```python
from build123d import *

# Parameters (mm, degrees)
SKETCH027_R             = 30
PAD006_DEPTH            = 13
SKETCH028_R             = 29
POCKET018_DEPTH         = 3.5
SKETCH029_R             = 27.5
PAD007_DEPTH            = 3.5
SKETCH031_W             = 32
SKETCH031_H             = 40
POCKET020_DEPTH         = 13
SKETCH032_W             = 5
SKETCH032_H             = 3
POCKET021_DEPTH         = 8
SKETCH033_R             = 2.25
POCKET022_DEPTH         = 20
SKETCH034_W             = 8
SKETCH034_H             = 5
POCKET023_DEPTH         = 10
SKETCH035_W             = 13.2
SKETCH035_H             = 7
POCKET024_DEPTH         = 9
SKETCH036_W             = 6.5
SKETCH036_H             = 7
POCKET025_DEPTH         = 5
SKETCH037_W             = 2
SKETCH037_H             = 13.2
PAD008_DEPTH            = 1
BODY005_PLACEMENT_ANGLE = 90


with BuildPart() as part:
    # Sketch027 → Pad006 (new body)
    with BuildSketch(Plane.XY):
        Circle(SKETCH027_R)
    extrude(amount=PAD006_DEPTH)

    # Sketch028 (on Face3 of Pad006) → Pocket018 (cut)
    with BuildSketch(Plane.XY.offset(13)):
        Circle(SKETCH028_R)
    extrude(amount=-POCKET018_DEPTH, mode=Mode.SUBTRACT)

    # Sketch029 (on Face5 of Pocket018) → Pad007 (join)
    with BuildSketch(Plane.XY.offset(9.5)):
        Circle(SKETCH029_R)
    extrude(amount=PAD007_DEPTH)

    # Sketch031 → Pocket020 (cut)
    with BuildSketch(Plane.XY.offset(13)):
        Rectangle(SKETCH031_W, SKETCH031_H)
    extrude(amount=-POCKET020_DEPTH, mode=Mode.SUBTRACT)

    # Sketch032 (on Face5 of Pocket020) → Pocket021 (cut)
    with BuildSketch(Plane(origin=(0, -20, 0), x_dir=(-1, 0, 0), z_dir=(0, 1, 0))):
        with Locations((0, 11.5)):
            Rectangle(SKETCH032_W, SKETCH032_H)
    extrude(amount=-POCKET021_DEPTH, mode=Mode.SUBTRACT)

    # Sketch033 (on Face9 of Pocket021) → Pocket022 (cut)
    with BuildSketch(Plane.XY.offset(13)):
        with Locations((-19.108778, -14.520833)):
            Circle(SKETCH033_R)
        with Locations((0, 24)):
            Circle(SKETCH033_R)
        with Locations((19.108778, -14.520833)):
            Circle(SKETCH033_R)
    extrude(amount=-POCKET022_DEPTH, mode=Mode.SUBTRACT)

    # Sketch034 (on Face2 of Pocket022) → Pocket023 (cut)
    with BuildSketch(Plane(origin=(0, 0, 0), x_dir=(1, 0, 0), z_dir=(0, 0, -1))):
        with Locations((0, 22.5)):
            Rectangle(SKETCH034_W, SKETCH034_H)
    extrude(amount=-POCKET023_DEPTH, mode=Mode.SUBTRACT)

    # Sketch035 (on Face10 of Pocket023) → Pocket024 (cut)
    with BuildSketch(Plane(origin=(16, 0, 0), x_dir=(0, -1, 0), z_dir=(-1, 0, 0))):
        with Locations((0, 3.5)):
            Rectangle(SKETCH035_W, SKETCH035_H)
    extrude(amount=-POCKET024_DEPTH, mode=Mode.SUBTRACT)

    # Sketch036 (on Face12 of Pocket024) → Pocket025 (cut)
    with BuildSketch(Plane(origin=(25, 0, 0), x_dir=(0, -1, 0), z_dir=(-1, 0, 0))):
        with Locations((0, 3.5)):
            Rectangle(SKETCH036_W, SKETCH036_H)
    extrude(amount=-POCKET025_DEPTH, mode=Mode.SUBTRACT)

    # Sketch037 (on Face7 of Pocket025) → Pad008 (join)
    with BuildSketch(Plane(origin=(0, 0, 7), x_dir=(1, 0, 0), z_dir=(0, 0, -1))):
        with Locations((17, 0)):
            Rectangle(SKETCH037_W, SKETCH037_H)
    extrude(amount=PAD008_DEPTH)


with BuildPart() as part_1:
    # Body005 placement: moved
    add(part.part.moved(Location((0, 0, 5))).rotate(Axis((0, 0, 5), (0, 0, 1)), BODY005_PLACEMENT_ANGLE))


solid = part_1.part
```
Check sheet for the modelled part. Datum: model origin and axes. Units: mm. A direction names the side the tool comes from. Round coordinates to 2 decimals unless told otherwise and drop trailing zeros. Order: outer loops, then holes, each group sorted by start corner. A loop starts at its lowest first (then second) coordinate and runs counter-clockwise, first axis right, second up. Notation, with made-up numbers: (11.5, 12.25) - (69.5, 12.25) arc R36 cw to (69.5, 46.25) - close; hole circle Ø8 at (9, 45.25). An arc over 180 degrees is marked (long way). Answer as CSV lines item,"result". Start each with the question number.
1) Section check B-B (x = 0). Record the cut outline in (y, z).
2) Draft check along X on faces 5 (the face through (25, 0, 10)), 6 (the face through (-2.2, 16.2, 18)). Enter one of: +X half, -X half, draft (parallel to the pull), parting line (faces both ways), or undercut.
3) Section check A-A (y = 0). Record the cut outline in (x, z), then the cut area to 4 significant figures.
4) Scan lines: probe 1 along X at (y, z) = (0, 17.1); probe 2 along X at (y, z) = (0, 10); probe 3 along Y at (x, z) = (-11, 14.75). Record each from-to range of solid material in increasing order.
5) Depth check by flat-ended pin: pin 1 (1.2 mm diameter, centred on x = 26, y = -1, fed in from +Z); pin 2 (4 mm diameter, centred on y = 2.5, z = 16.5, fed in from +X); pin 3 (5 mm diameter, centred on y = 11.5, z = 10.5, fed in from +X); pin 4 (4 mm diameter, centred on x = 14.52, y = -19.11, fed in from -Z). Enter the tip coordinate at first touch or a pass-through.
6) Tool access check on faces 1 (the face through (3.25, 27, 8)), 2 (the face through (5, 25, 9)), 3 (the face through (20, 9, 12)), 4 (the face through (26, 0, 15)). Record the directions out of +Z, -Z, +X, -X, +Y, -Y that give a thin tool (end or side, any length) a straight path to the whole face; none if there is none.
7) Section check D-D (z = 13.5). Record the cut outline in (x, y), then the cut area to 3 significant figures.
8) Section check C-C (z = 8.25). Record the cut outline in (x, y), then the cut area to 3 significant figures.
Determined:
1,outline,"(-30, 5) - (-16, 5) - (-16, 18) - (-27.5, 18) - (-27.5, 14.5) - (-29, 14.5) - (-29, 18) - (-30, 18) - close; (16, 11) - (18, 11) - (18, 12) - (30, 12) - (30, 18) - (29, 18) - (29, 14.5) - (27.5, 14.5) - (27.5, 18) - (16, 18) - close"
2,face 5,"undercut"
2,face 6,"draft"
3,outline,"(-30, 5) - (-26.25, 5) - (-26.25, 18) - (-27.5, 18) - (-27.5, 14.5) - (-29, 14.5) - (-29, 18) - (-30, 18) - close; (-21.75, 5) - (-20, 5) - (-20, 18) - (-21.75, 18) - close; (25, 5) - (30, 5) - (30, 18) - (29, 18) - (29, 14.5) - (27.5, 14.5) - (27.5, 15) - (25, 15) - close"
3,area,"118.5 mm^2"
4,probe 1,"-30 to -29, -27.5 to -26.25, -21.75 to -20, 29 to 30"
4,probe 2,"-30 to -26.25, -21.75 to -20, 25 to 30"
4,probe 3,"-27.91 to -26.83, -25.2 to -16, 16 to 25.2, 26.83 to 27.91"
5,pin 1,"z = 15"
5,pin 2,"x = 30"
5,pin 3,"x = 28.62"
5,pin 4,"through"
6,face 1,"-Z, +Y"
6,face 2,"-Z"
6,face 3,"+Z, -Z"
6,face 4,"+Z"
7,outline,"circle Ø60 at (0, 0); hole circle Ø4.5 at (-24, 0); hole (-20, -16) - (20, -16) - (20, -4) - (25, -4) - (25, 4) - (20, 4) - (20, 16) - (-20, 16) - close; hole circle Ø4.5 at (14.52, -19.11); hole circle Ø4.5 at (14.52, 19.11)"
7,area,"1,460 mm^2"
8,outline,"(-20, -16) - (-20, 16) - (-6.6, 16) - (-6.6, 25) - (-3.25, 25) - (-3.25, 29.82) arc R30 ccw (long way) to (3.25, 29.82) - (3.25, 25) - (6.6, 25) - (6.6, 16) - (20, 16) - (20, 4) - (25, 4) - (25, -4) - (20, -4) - (20, -16) - close; hole circle Ø4.5 at (-24, 0); hole circle Ø4.5 at (14.52, -19.11); hole circle Ø4.5 at (14.52, 19.11)"
8,area,"1,310 mm^2"
